Can you work these out from the model? Positions are in its coordinate system, mm. Give positions to 0.01 mm unless a question says otherwise; leave off trailing zeros. Write each loop counter-clockwise with the first axis right and the second up, starting at its lowest first coordinate (ties: lowest second). Pieces come first, ordered by that corner, then holes. Notation, with made-up numbers: M 59,79 L 70,79 A22 cw 70,109 Z; hole C 65.25,14 d5. An arc over 180 degrees is marked long. Write each question's results on one line, items separated by ' | '.
from build123d import *

# Parameters (mm, degrees)
SKETCH1_W           = 1040
SKETCH1_H           = 50.8
BOSS_EXTRUDE1_DEPTH = 38.1
SKETCH7_R           = 1.5
CUT_EXTRUDE14_DEPTH = 5
CUT_EXTRUDE15_DEPTH = 10
CUT_EXTRUDE16_DEPTH = 4.7625
SKETCH2_W           = 4
SKETCH2_H           = 2
CUT_EXTRUDE18_DEPTH = 39.1
HOLE2_AT_2_COUNT    = 2
HOLE2_AT_2_PITCH    = 7.294
HOLE2_AT_3_COUNT    = 2
HOLE2_AT_3_PITCH    = 14.588
HOLE2_AT_4_COUNT    = 2
HOLE2_AT_4_PITCH    = 20.948
HOLE2_AT_5_COUNT    = 2
HOLE2_AT_5_PITCH    = 27.308
HOLE2_AT_6_COUNT    = 2
HOLE2_AT_6_PITCH    = 32.42


with BuildPart() as part:
    # Sketch1 → Boss-Extrude1 (new body)
    with BuildSketch(Plane(origin=(0, 0, 0), x_dir=(1, 0, 0), z_dir=(0, 1, 0))):
        with Locations((520, 25.4)):
            Rectangle(SKETCH1_W, SKETCH1_H)
    extrude(amount=BOSS_EXTRUDE1_DEPTH)

    # Sketch7 → Cut-Extrude14 (cut)
    with BuildSketch(Plane(origin=(0, 38.1, 0), x_dir=(1, 0, 0), z_dir=(0, 1, 0))):
        with Locations(Location((400, 6.513, 0), (0, 0, 270))):  # turned: the seam where the file's is
            Circle(SKETCH7_R)
        with Locations(Location((160, 6.513, 0), (0, 0, 270))):  # turned: the seam where the file's is
            Circle(SKETCH7_R)
        with Locations(Location((870, 6.513, 0), (0, 0, 270))):  # turned: the seam where the file's is
            Circle(SKETCH7_R)
        with Locations(Location((630, 6.513, 0), (0, 0, 270))):  # turned: the seam where the file's is
            Circle(SKETCH7_R)
        with Locations(Location((170, 10.725, 0), (0, 0, 270))):  # turned: the seam where the file's is
            Circle(SKETCH7_R)
        with Locations(Location((30, 6.513, 0), (0, 0, 270))):  # turned: the seam where the file's is
            Circle(SKETCH7_R)
        with Locations(Location((40, 10.725, 0), (0, 0, 270))):  # turned: the seam where the file's is
            Circle(SKETCH7_R)
        with Locations(Location((1000, 6.513, 0), (0, 0, 270))):  # turned: the seam where the file's is
            Circle(SKETCH7_R)
        with Locations(Location((410, 10.725, 0), (0, 0, 270))):  # turned: the seam where the file's is
            Circle(SKETCH7_R)
        with Locations(Location((1010, 10.725, 0), (0, 0, 270))):  # turned: the seam where the file's is
            Circle(SKETCH7_R)
        with Locations(Location((640, 10.725, 0), (0, 0, 270))):  # turned: the seam where the file's is
            Circle(SKETCH7_R)
        with Locations(Location((880, 10.725, 0), (0, 0, 270))):  # turned: the seam where the file's is
            Circle(SKETCH7_R)
    extrude(amount=-CUT_EXTRUDE14_DEPTH, mode=Mode.SUBTRACT)

    # Sketch8 → Cut-Extrude15 (cut)
    with BuildSketch(Plane.XZ):
        with BuildLine():
            Line((12, -44.8), (1028, -44.8))
            ThreePointArc((1028, -44.8), (1032.242640687, -43.042640687), (1034, -38.8))
            Line((1034, -38.8), (1034, -12))
            ThreePointArc((1034, -12), (1032.242640687, -7.757359313), (1028, -6))
            Line((1028, -6), (12, -6))
            ThreePointArc((12, -6), (7.757359313, -7.757359313), (6, -12))
            Line((6, -12), (6, -38.8))
            ThreePointArc((6, -38.8), (7.757359313, -43.042640687), (12, -44.8))
        make_face()
    extrude(amount=-CUT_EXTRUDE15_DEPTH, mode=Mode.SUBTRACT)

    # Sketch8_3 → Cut-Extrude16 (cut)
    with BuildSketch(Plane.XZ):
        with BuildLine():
            Line((9, -47.8), (1031, -47.8))
            ThreePointArc((1031, -47.8), (1035.242640687, -46.042640687), (1037, -41.8))
            Line((1037, -41.8), (1037, -9))
            ThreePointArc((1037, -9), (1035.242640687, -4.757359313), (1031, -3))
            Line((1031, -3), (9, -3))
            ThreePointArc((9, -3), (4.757359313, -4.757359313), (3, -9))
            Line((3, -9), (3, -41.8))
            ThreePointArc((3, -41.8), (4.757359313, -46.042640687), (9, -47.8))
        make_face()
    extrude(amount=-CUT_EXTRUDE16_DEPTH, mode=Mode.SUBTRACT)

    # Sketch2 → Cut-Extrude18 (cut, through all)
    with BuildSketch(Plane(origin=(0, 38.1, 0), x_dir=(1, 0, 0), z_dir=(0, 1, 0))):
        with Locations((45, 1)):
            Rectangle(SKETCH2_W, SKETCH2_H)
        with Locations((282.5, 1)):
            Rectangle(SKETCH2_W, SKETCH2_H)
        with Locations((520, 1)):
            Rectangle(SKETCH2_W, SKETCH2_H)
        with Locations((757.5, 1)):
            Rectangle(SKETCH2_W, SKETCH2_H)
        with Locations((995, 1)):
            Rectangle(SKETCH2_W, SKETCH2_H)
    extrude(amount=-CUT_EXTRUDE18_DEPTH, mode=Mode.SUBTRACT)

    # Sketch12 → 1_8 NPT Tapped Hole2 (revolve, cut)
    with BuildSketch(Plane(origin=(1040, 12, -25.4), x_dir=(0, 0, -1), z_dir=(0, 1, 0))):
        Polygon((0, 0), (0, 27.533468714), (4.2164, 25), (4.2164, 6.92), (4.537398933, 6.92), (4.744593, 0), align=None)
    revolve(axis=Axis((1046.35, 12, -25.4), (-1, 0, 0)), mode=Mode.SUBTRACT)

    # Sketch14 → 1_8 NPT Tapped Hole3 (revolve, cut)
    with BuildSketch(Plane(origin=(0, 12, -25.4), x_dir=(0, 0, 1), z_dir=(0, 1, 0))):
        Polygon((0, 0), (0, 27.533468714), (4.2164, 25), (4.2164, 6.92), (4.537398933, 6.92), (4.744593, 0), align=None)
    revolve(axis=Axis((-6.35, 12, -25.4), (1, 0, 0)), mode=Mode.SUBTRACT)

    # Sketch26 → Hole2 (revolve, cut)
    with BuildSketch(Plane(origin=(15, 10, -42.533), x_dir=(0, 0, -1), z_dir=(1, 0, 0))):
        Polygon((0, 0), (0, 28.1), (0.79375, 28.1), (0.79375, 20.953866233), (2.38125, 20), (2.38125, 0), align=None)
    hole2 = revolve(axis=Axis((15, 3.869976101, -42.533), (0, 1, 0)), mode=Mode.SUBTRACT)

    # Hole2 at 2: Hole2 ×2
    with Locations(*[(0, 0, i * HOLE2_AT_2_PITCH) for i in range(1, HOLE2_AT_2_COUNT)]):
        add(hole2, mode=Mode.SUBTRACT)

    # Hole2 at 3: Hole2 ×2
    with Locations(*[(0, 0, i * HOLE2_AT_3_PITCH) for i in range(1, HOLE2_AT_3_COUNT)]):
        add(hole2, mode=Mode.SUBTRACT)

    # Hole2 at 4: Hole2 ×2
    with Locations(*[(0, 0, i * HOLE2_AT_4_PITCH) for i in range(1, HOLE2_AT_4_COUNT)]):
        add(hole2, mode=Mode.SUBTRACT)

    # Hole2 at 5: Hole2 ×2
    with Locations(*[(0, 0, i * HOLE2_AT_5_PITCH) for i in range(1, HOLE2_AT_5_COUNT)]):
        add(hole2, mode=Mode.SUBTRACT)

    # Hole2 at 6: Hole2 ×2
    with Locations(*[(0, 0, i * HOLE2_AT_6_PITCH) for i in range(1, HOLE2_AT_6_COUNT)]):
        add(hole2, mode=Mode.SUBTRACT)


solid = part.part
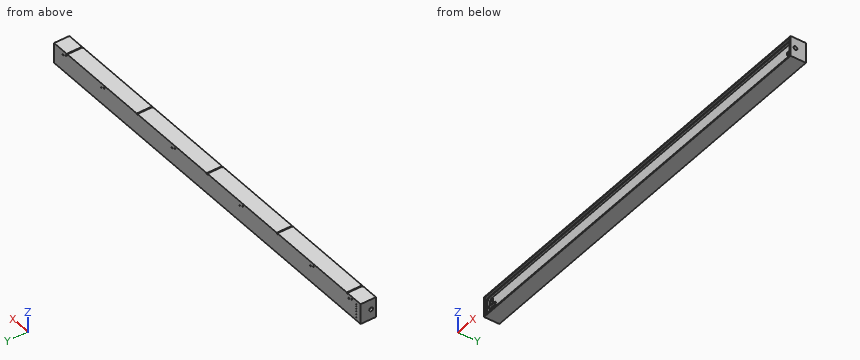
Item 1: I want a section at A-A, the plane x = 909.5. Please give me the cut outline in (y, z).
Geometry says:
outline: M 0,-50.8 L 38.1,-50.8 L 38.1,0 L 0,0 L 0,-3 L 4.76,-3 L 4.76,-6 L 10,-6 L 10,-44.8 L 4.76,-44.8 L 4.76,-47.8 L 0,-47.8 Z
Item 2: If I drill on line 1 (X direction, y = 5.5, z = -27.5); line 2 (Z direction, x = 1010, y = 37.1) (3 decimals); line 3 (X direction, y = 17.5, z = -36), over which ranges is the centre line in solid material (lowest first)? Write a range as from..to.
Geometry says:
line 1: x = 0..6, 1034..1040 | line 2: z = -50.8..-12.225, -9.225..0 | line 3: x = 0..12.74, 17.26..1040
Item 3: I'm going to push flat-ended pins straight in: pin 1 (1 mm diameter, centred on x = 934, z = -24, fed in from -Y); pin 2 (4 mm diameter, centred on x = 630, z = -6.513, fed in from -Y); pin 3 (2 mm diameter, centred on x = 282.5, y = 22.5, fed in from +Z). Where does each tip first touch, or does it pass through?
Geometry says:
pin 1: stops at y = 10 | pin 2: stops at y = 4.76 | pin 3: stops at z = -2
